```python
from build123d import *

# Parameters (mm, degrees)
SKETCH1_R               = 2.5
BOSS_EXTRUDE1_DEPTH     = 9.1
CUT_EXTRUDE1_DEPTH      = 20.618613611
CUT_EXTRUDE1_DEPTH_BACK = 20.618613611
SKETCH4_W               = 5.29751814
SKETCH4_H               = 11.035514004
SKETCH5_R               = 5
BOSS_EXTRUDE2_DEPTH     = 10
CUT_EXTRUDE2_DEPTH      = 28.779051493
CUT_EXTRUDE2_DEPTH_BACK = 8
SKETCH6_R               = 4


with BuildPart() as part:
    # Sketch1 → Boss-Extrude1 (new body)
    with BuildSketch(Plane.XY):
        with Locations((0, -0.210420065)):
            Circle(SKETCH1_R)
    extrude(amount=BOSS_EXTRUDE1_DEPTH)

    # Sketch3 → Revolve1 (revolve)
    with BuildSketch(Plane(origin=(0, 0, 0), x_dir=(0, 0, -1), z_dir=(1, 0, 0))):
        with BuildLine():
            Line((-13.3, -5), (-13.3, 5))
            ThreePointArc((-13.3, 5), (-8.3, 0), (-13.3, -5))
        make_face()
    revolve(axis=Axis((0, -5, 13.3), (0, 1, 0)))

    # Sketch4 → Cut-Extrude1 (cut, two sides: drawn at the far end of the back side and taken through both)
    with BuildSketch(Plane(origin=(0, 0, 0), x_dir=(0, 0, -1), z_dir=(1, 0, 0)).offset(-CUT_EXTRUDE1_DEPTH_BACK)):
        with Locations((-19.512781414, 0.215959178)):
            Rectangle(SKETCH4_W, SKETCH4_H)
    extrude(amount=CUT_EXTRUDE1_DEPTH + CUT_EXTRUDE1_DEPTH_BACK, mode=Mode.SUBTRACT)

    # Sketch5 → Boss-Extrude2 (add)
    with BuildSketch(Plane(origin=(0, 0, 0), x_dir=(-1, 0, 0), z_dir=(0, 0, -1))):
        Circle(SKETCH5_R)
    extrude(amount=BOSS_EXTRUDE2_DEPTH)

    # Sketch6 → Cut-Extrude2 (cut, two sides: drawn at the far end of the back side and taken through both)
    with BuildSketch(Plane(origin=(0, 0, -10), x_dir=(-1, 0, 0), z_dir=(0, 0, -1)).offset(-CUT_EXTRUDE2_DEPTH_BACK)):
        with Locations(Location((0, 0, 0), (0, 0, 180))):
            Circle(SKETCH6_R)
    extrude(amount=CUT_EXTRUDE2_DEPTH + CUT_EXTRUDE2_DEPTH_BACK, mode=Mode.SUBTRACT)


solid = part.part
```
Could you check a few things on this model? Use its own coordinates, in mm. A direction names the side the tool comes from. Coordinates: 2 decimals unless noted, no trailing zeros. Order: outer loops, then holes, each group sorted by start corner. A loop starts at its lowest first (then second) coordinate and runs counter-clockwise, first axis right, second up. Notation, with made-up numbers: M 89,-31.75 L 123,-31.75 A21 cw 123,-27.75 Z; hole C -20,5 d3. An arc over 180 degrees is marked long. Use a Markdown table: item, result. Add a question column.
Q1. I want a section at A-A on x = 3. List the corners of the cut face in (y, z) for me, then the cut area to 3 significant figures.
Q2. I want a section at B-B on y = 4.75. List the corners of the cut face in (x, z) for me, then the cut area to 3 significant figures.
Q3. I want a section at D-D on y = 1. List the corners of the cut face in (x, z) for me, then the cut area to 3 significant figures.
Q4. I'm going to push flat-ended pins straight in: pin 1 (2 mm diameter, centred on y = 3.5, z = 0, fed in from +X); pin 2 (1.5 mm diameter, centred on x = -1.5, z = 1, fed in from -Y); pin 3 (1 mm diameter, centred on y = 2.5, z = 7.5, fed in from -X). Where does each tip first touch, or does it pass through?
Q5. I want a section at C-C on z = -7. List the corners of the cut face in (x, y) for me, then the cut area to 3 significant figures.
Q6. Which directions (+Z, -Z, +X, -X, +Y, -Y) give clear straight access to the entire face, cutting with the end or side of a thin tool? Please do faces 1 (the flat face through (-1, 2.3, 0)), 2 (the flat face through (0, 0, -2)).
Q7. If I drill on L1, parallel to Y at x = 0, z = -5.25; L2, parallel to Z at x = -1.5, y = 3; L3, parallel to Z at x = 1, y = -4.5, over which ranges is the centre line in solid material (lowest first)?
Q8. We'd pull the mould along X, two halves only. Please class faces 3 (the flat face through (0, 0, 16.864)), 4 (the cylindrical face through (1.08, -4.88, -4.93)), 5 (the cylindrical face through (-0.867, 3.905, -5.944)): pulls with the +X half, pulls with the -X half, needs draft (parallel to the pull), parting line crosses it, or undercut.
Checked values:
| question | item | result |
|---|---|---|
| 1 | outline | M -4,-10 L -2.65,-10 L -2.65,-2 L 2.65,-2 L 2.65,-10 L 4,-10 L 4,0 L -4,0 Z; M -1.82,16.86 A4 ccw long 1.82,16.86 Z |
| 1 | area | 86.9 mm² |
| 2 | outline | M -1.56,-10 L 1.56,-10 L 1.56,0 L -1.56,0 Z; C 0,13.3 d3.12 |
| 2 | area | 38.9 mm² |
| 3 | outline | M -4.9,-10 L -3.87,-10 L -3.87,-2 L 3.87,-2 L 3.87,-10 L 4.9,-10 L 4.9,0 L 2.19,0 L 2.19,8.92 A4.9 ccw 3.36,16.86 L -3.36,16.86 A4.9 ccw -2.19,8.92 L -2.19,0 L -4.9,0 Z |
| 3 | area | 143 mm² |
| 4 | pin 1 | x = 4.33 |
| 4 | pin 2 | y = -2.6 |
| 4 | pin 3 | x = -1.17 |
| 5 | outline | C 0,0 d10; hole C 0,0 d8 |
| 5 | area | 28.3 mm² |
| 6 | face 1 | none |
| 6 | face 2 | -Z |
| 7 | L1 | -5 to -4, 4 to 5 |
| 7 | L2 | -2 to 0, 9.59 to 16.86 |
| 7 | L3 | -10 to 0, 11.36 to 15.24 |
| 8 | face 3 | needs draft |
| 8 | face 4 | parting line crosses it |
| 8 | face 5 | undercut |
